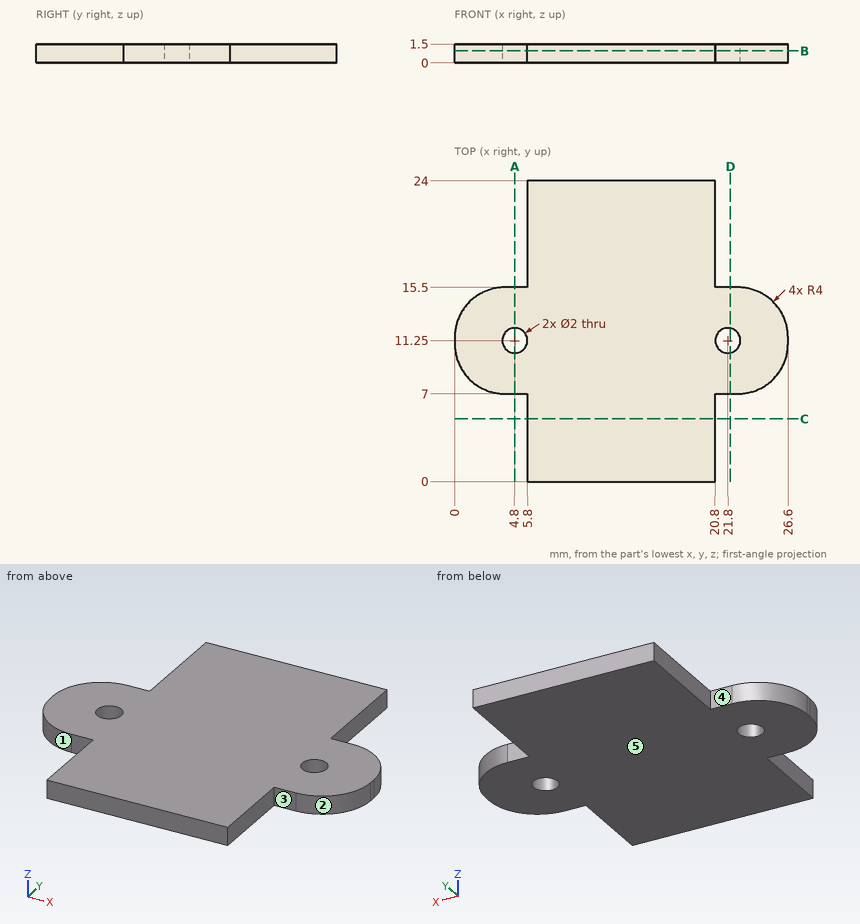
The figure shows three views and two pictorial views of one solid part (mm, origin at its lowest corner). Answer the questions. A direction names the side the tool comes from. Round coordinates to 2 decimals unless told otherwise and drop trailing zeros. Write each loop counter-clockwise with the first axis right and the second up, starting at its lowest first coordinate (ties: lowest second). Pieces come first, ordered by that corner, then holes. Notation, with made-up numbers: M -40,-16.5 L -16,-16.5 A22 ccw -16,16.5 Z; hole C 76,19.5 d6. An arc over 180 degrees is marked long. Write each question's results on one line, items separated by ' | '. Start each with the question number.
(1) The part is cut by section C-C, the plane y = 5. Write down the section's boundary in (x, z).
(2) The part is cut by section A-A, the plane x = 4.8. Write down the section's boundary in (y, z), and give its area (3 significant figures).
(3) Each of these flat-tipped pins is pushed along its axis until it touches: P1, Ø1.5, axis at x = 4.5, y = 3, coming from the +Z side; P2, Ø0.8, axis at x = 21.5, z = 0.5, coming from the -Y side; P3, Ø0.8, axis at x = 4.5, z = 1, coming from the +Y side; P4, Ø4, axis at x = 12.5, y = 14, coming from the -Z side. Where does it stop, or does it pass through?
(4) The part is cut by section B-B, the plane z = 0.95. Write down the section's boundary in (x, y).
(5) For the marked faces 4 and 5, determine the directions among +Z, -Z, +X, -X, +Y, -Y from which every point of the face is accessible in a straight line to the end or side of a thin tool.
(6) Find the intervals of material crossed by line 1 (Y direction, x = 21.8, z = 0.9); line 2 (X direction, y = 2, z = 0.7); line 3 (X direction, y = 8.75, z = 1.15), in increasing order.
(7) The part is cut by section D-D, the plane x = 22. Write down the section's boundary in (y, z).
(8) Determine the mould class of the marked faces 1, 2 and 3 for opening direction X: +X half, -X half, draft (parallel to the pull), parting line (faces both ways), or undercut.
Worked answers:
1) outline: M 5.8,0 L 20.8,0 L 20.8,1.5 L 5.8,1.5 Z
2) outline: M 7,0 L 10.25,0 L 10.25,1.5 L 7,1.5 Z; M 12.25,0 L 15.5,0 L 15.5,1.5 L 12.25,1.5 Z | area: 9.75 mm²
3) P1: passes through | P2: stops at y = 7 | P3: stops at y = 15.5 | P4: stops at z = 0
4) outline: M 0,11 A4 ccw 4,7 L 5.8,7 L 5.8,0 L 20.8,0 L 20.8,7 L 22.6,7 A4 ccw 26.6,11 L 26.6,11.5 A4 ccw 22.6,15.5 L 20.8,15.5 L 20.8,24 L 5.8,24 L 5.8,15.5 L 4,15.5 A4 ccw 0,11.5 Z; hole C 4.8,11.25 d2; hole C 21.8,11.25 d2
5) face 4: +Z, -Z, -X, +Y | face 5: -Z, +X, -X, +Y, -Y
6) line 1: y = 7 to 10.25, 12.25 to 15.5 | line 2: x = 5.8 to 20.8 | line 3: x = 0.69 to 25.91
7) outline: M 7,0 L 10.27,0 L 10.27,1.5 L 7,1.5 Z; M 12.23,0 L 15.5,0 L 15.5,1.5 L 12.23,1.5 Z
8) face 1: -X half | face 2: +X half | face 3: draft
